Verification items for the finished model (mm, model axes). Face numbers are marked on the shaded views. A direction names the side the tool comes from. Coordinates: 2 decimals unless noted, no trailing zeros. Loops run counter-clockwise (first coordinate to the right, second up) from the corner with the lowest first, then second, coordinate; pieces in that order, holes last. Notation, with made-up numbers: (10, 81) - (28, 81) arc R20 cw to (28, 100) - close; hole circle Ø8 at (71.25, 5). An arc over 180 degrees is marked (long way). One line per item, written item: value. Start each with the question number.
(1) Thickness scan on probe 1 along X at (y, z) = (2.25, -33.5); probe 2 along Z at (x, y) = (-22, 4); probe 3 along Z at (x, y) = (-21.25, 1). Record the ranges inside material, lowest first. Write a range as [from, to].
(2) Section check B-B (y = 1.75). Record the boundary of the cut face in (x, z), plus the area to 3 significant figures.
(3) Section check A-A (z = -24.5). Record the boundary of the cut face in (x, y), plus the area to 3 significant figures.
(4) Gauge pin test, flat ends, axial feed: P1, Ø3, axis at x = -8, z = -34, coming from the +Y side; P2, Ø2.5, axis at x = -7.82, z = -13.46, coming from the +Y side; P3, Ø1.8, axis at x = -14.82, y = 11, coming from the +Z side; P4, Ø5.5, axis at y = 3, z = -23, coming from the +X side. Record the tip position at first contact, or that the pin passes through.
(5) Section check D-D (z = -14). Record the boundary of the cut face in (x, y).
(6) Set-up check for the marked faces 1, 2, 3, 4 and 5: record each of +Z, -Z, +X, -X, +Y, -Y from which the full face is reachable in a straight line by a thin tool's end or side.
(7) Section check C-C (x = -14.25). Record the boundary of the cut face in (y, z), plus the area to 3 significant figures.
```python
from build123d import *

# Parameters (mm, degrees)
SKETCH_1_R          = 1
EXTRUDE_1_DEPTH     = 5
SKETCH_7_R          = 1.5
EXTRUDE_3_DEPTH     = 30
SKETCH_8_R          = 2
CUT_EXTRUDE_1_DEPTH = 2


with BuildPart() as part:
    # 草图1 → 凸台-拉伸1 (new body)
    with BuildSketch(Plane(origin=(0, 0, 0), x_dir=(1, 0, 0), z_dir=(0, 1, 0))):
        with BuildLine():
            Line((-21.819389518, 18.45581381), (-20.819389518, 18.45581381))
            ThreePointArc((-20.819389518, 18.45581381), (-20.112282737, 18.748707029), (-19.819389518, 19.45581381))
            Line((-19.819389518, 19.45581381), (-19.819389518, 27.45581381))
            ThreePointArc((-19.819389518, 27.45581381), (-20.112282737, 28.162920591), (-20.819389518, 28.45581381))
            Line((-20.819389518, 28.45581381), (-21.819389518, 28.45581381))
            ThreePointArc((-21.819389518, 28.45581381), (-26.819389518, 33.45581381), (-21.819389518, 38.45581381))
            Line((-21.819389518, 38.45581381), (-7.819389518, 38.45581381))
            ThreePointArc((-7.819389518, 38.45581381), (-2.819389518, 33.45581381), (-7.819389518, 28.45581381))
            Line((-7.819389518, 28.45581381), (-8.819389518, 28.45581381))
            ThreePointArc((-8.819389518, 28.45581381), (-9.526496299, 28.162920591), (-9.819389518, 27.45581381))
            Line((-9.819389518, 27.45581381), (-9.819389518, 19.45581381))
            ThreePointArc((-9.819389518, 19.45581381), (-9.526496299, 18.748707029), (-8.819389518, 18.45581381))
            Line((-8.819389518, 18.45581381), (-7.819389518, 18.45581381))
            ThreePointArc((-7.819389518, 18.45581381), (-2.819389518, 13.45581381), (-7.819389518, 8.45581381))
            Line((-7.819389518, 8.45581381), (-21.819389518, 8.45581381))
            ThreePointArc((-21.819389518, 8.45581381), (-26.819389518, 13.45581381), (-21.819389518, 18.45581381))
        make_face()
        with Locations(Location((-21.819389518, 13.45581381, 0), (0, 0, 270))):
            Circle(SKETCH_1_R, mode=Mode.SUBTRACT)
        with Locations(Location((-7.819389518, 13.45581381, 0), (0, 0, 270))):
            Circle(SKETCH_1_R, mode=Mode.SUBTRACT)
        with Locations(Location((-21.819389518, 33.45581381, 0), (0, 0, 270))):
            Circle(SKETCH_1_R, mode=Mode.SUBTRACT)
        with Locations(Location((-7.819389518, 33.45581381, 0), (0, 0, 270))):
            Circle(SKETCH_1_R, mode=Mode.SUBTRACT)
    extrude(amount=EXTRUDE_1_DEPTH)

    # 草图7 → 凸台-拉伸3 (add)
    with BuildSketch(Plane.XY.offset(-8.45581381)):
        with BuildLine():
            Line((-17.819389518, 11), (-17.819389518, 5))
            Line((-17.819389518, 5), (-11.819389518, 5))
            Line((-11.819389518, 5), (-11.819389518, 11))
            ThreePointArc((-11.819389518, 11), (-14.819389518, 14), (-17.819389518, 11))
        make_face()
        with Locations((-14.819389518, 11)):
            Circle(SKETCH_7_R, mode=Mode.SUBTRACT)
    extrude(amount=-EXTRUDE_3_DEPTH)

    # 草图8 → 切除-拉伸1 (cut)
    with BuildSketch(Plane(origin=(0, 5, 0), x_dir=(1, 0, 0), z_dir=(0, 1, 0))):
        with Locations(Location((-21.819389518, 33.45581381, 0), (0, 0, 270))):
            Circle(SKETCH_8_R)
        with Locations(Location((-7.819389518, 33.45581381, 0), (0, 0, 270))):
            Circle(SKETCH_8_R)
        with Locations(Location((-21.819389518, 13.45581381, 0), (0, 0, 270))):
            Circle(SKETCH_8_R)
        with Locations(Location((-7.819389518, 13.45581381, 0), (0, 0, 270))):
            Circle(SKETCH_8_R)
    extrude(amount=-CUT_EXTRUDE_1_DEPTH, mode=Mode.SUBTRACT)


solid = part.part
```
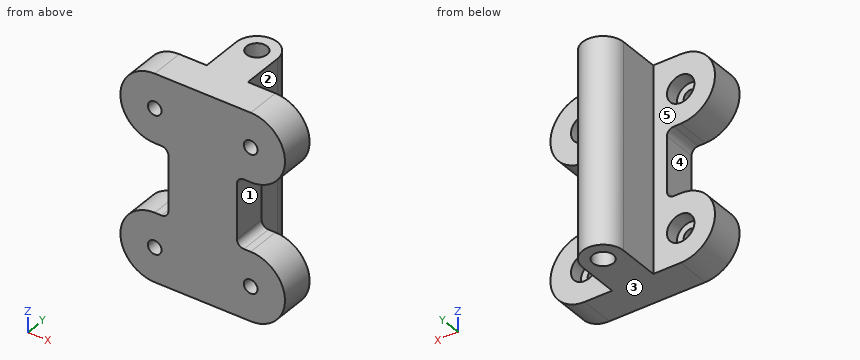
Responses:
1. probe 1: x = [-26.82, -22.82], [-20.82, -8.82], [-6.82, -2.82]
1. probe 2: z = [-38.45, -35.45], [-31.46, -28.46], [-18.45, -15.45], [-11.46, -8.46]
1. probe 3: z = [-38.46, -34.28], [-32.63, -28.46], [-18.46, -14.28], [-12.63, -8.46]
2. outline: (-21.82, -38.46) - (-7.82, -38.46) arc R5 ccw to (-7.82, -28.46) - (-8.82, -28.46) arc R1 cw to (-9.82, -27.46) - (-9.82, -19.46) arc R1 cw to (-8.82, -18.46) - (-7.82, -18.46) arc R5 ccw to (-7.82, -8.46) - (-21.82, -8.46) arc R5 ccw to (-21.82, -18.46) - (-20.82, -18.46) arc R1 cw to (-19.82, -19.46) - (-19.82, -27.46) arc R1 cw to (-20.82, -28.46) - (-21.82, -28.46) arc R5 ccw to start; hole circle Ø2 at (-21.82, -33.46); hole circle Ø2 at (-21.82, -13.46); hole circle Ø2 at (-7.82, -33.46); hole circle Ø2 at (-7.82, -13.46)
2. area: 525 mm²
3. outline: (-19.82, 0) - (-9.82, 0) - (-9.82, 5) - (-11.82, 5) - (-11.82, 11) arc R3 ccw to (-17.82, 11) - (-17.82, 5) - (-19.82, 5) - close; hole circle Ø3 at (-14.82, 11)
3. area: 93.1 mm²
4. P1: stops at y = 5
4. P2: stops at y = 3
4. P3: passes through
4. P4: stops at x = -9.82
5. outline: (-26.79, 0) - (-22.66, 0) - (-22.66, 3) - (-23.74, 3) - (-23.74, 5) - (-26.79, 5) - close; (-20.98, 0) - (-8.66, 0) - (-8.66, 3) - (-9.74, 3) - (-9.74, 5) - (-11.82, 5) - (-11.82, 11) arc R3 ccw to (-17.82, 11) - (-17.82, 5) - (-19.89, 5) - (-19.89, 3) - (-20.98, 3) - close; (-6.98, 0) - (-2.85, 0) - (-2.85, 5) - (-5.89, 5) - (-5.89, 3) - (-6.98, 3) - close; hole circle Ø3 at (-14.82, 11)
6. face 1: +X, +Y, -Y
6. face 2: +Z, -Z, +X, +Y
6. face 3: -Z, +X, -X, +Y, -Y
6. face 4: -X, +Y, -Y
6. face 5: +Z, -Z, -X, +Y
7. outline: (0, -38.46) - (9.61, -38.46) - (9.61, -8.46) - (0, -8.46) - close; (12.39, -38.46) - (13.95, -38.46) - (13.95, -8.46) - (12.39, -8.46) - close
7. area: 335 mm²
